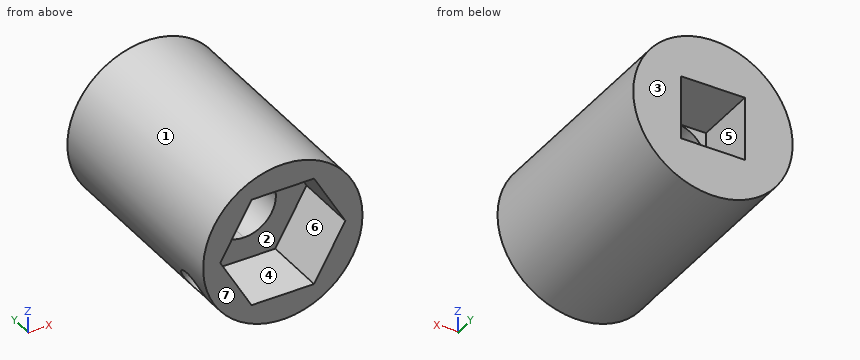
```python
from build123d import *

# Parameters (mm, degrees)
F0_R     = 63.5
F1_DEPTH = 127
F3_DEPTH = 127.001
F4_DEPTH = 50.8
F5_R     = 63.5
F6_DEPTH = 50.8
F7_R     = 13.4769297295
F8_DEPTH = 43.5797324345


with BuildPart() as f1:
    # F0 (on Front) → F1 (new body)
    with BuildSketch(Plane.XZ):
        Circle(F0_R)
    extrude(amount=F1_DEPTH)

    # F2 (on Front) → F3 (cut, through all)
    with BuildSketch(Plane.XZ):
        with BuildLine():
            ThreePointArc((25.4, 0), (17.9605122594, 17.9605122249), (4.89e-08, 25.4))
            ThreePointArc((4.89e-08, 25.4), (-17.9605122127, 17.9605122716), (-25.4, 3.44e-08))
            ThreePointArc((-25.4, 3.44e-08), (-17.9605122437, -17.9605122406), (3.01e-08, -25.4))
            ThreePointArc((3.01e-08, -25.4), (17.9605122528, -17.9605122315), (25.4, 0))
        make_face()
    extrude(amount=F3_DEPTH, mode=Mode.SUBTRACT)

    # F2 (on Front) → F4 (cut)
    with BuildSketch(Plane.XZ):
        with BuildLine():
            Line((4.89e-08, 25.4), (-25.4, 25.4))
            Line((-25.4, 25.4), (-25.4, 3.44e-08))
            ThreePointArc((-25.4, 3.44e-08), (-17.9605122127, 17.9605122716), (4.89e-08, 25.4))
        make_face()
        with BuildLine():
            Line((25.4, 25.4), (4.89e-08, 25.4))
            ThreePointArc((4.89e-08, 25.4), (17.9605122594, 17.9605122249), (25.4, 0))
            Line((25.4, 0), (25.4, 25.4))
        make_face()
        with BuildLine():
            ThreePointArc((25.4, 0), (17.9605122594, 17.9605122249), (4.89e-08, 25.4))
            ThreePointArc((4.89e-08, 25.4), (-17.9605122127, 17.9605122716), (-25.4, 3.44e-08))
            ThreePointArc((-25.4, 3.44e-08), (-17.9605122437, -17.9605122406), (3.01e-08, -25.4))
            ThreePointArc((3.01e-08, -25.4), (17.9605122528, -17.9605122315), (25.4, 0))
        make_face()
        with BuildLine():
            ThreePointArc((3.01e-08, -25.4), (-17.9605122437, -17.9605122406), (-25.4, 3.44e-08))
            Line((-25.4, 3.44e-08), (-25.4, -25.4))
            Line((-25.4, -25.4), (3.01e-08, -25.4))
        make_face()
        with BuildLine():
            Line((25.4, -25.4), (25.4, 0))
            ThreePointArc((25.4, 0), (17.9605122528, -17.9605122315), (3.01e-08, -25.4))
            Line((3.01e-08, -25.4), (25.4, -25.4))
        make_face()
    extrude(amount=F4_DEPTH, mode=Mode.SUBTRACT)

    # F5 (on face) → F6 (join)
    with BuildSketch(Plane.XZ.offset(127)):
        Circle(F5_R)
        Polygon((-49.8413562896, 0), (-24.9206781448, 43.1638807058), (24.9206781448, 43.1638807058), (49.8413562896, 0), (24.9206781448, -43.1638807058), (-24.9206781448, -43.1638807058), align=None, mode=Mode.SUBTRACT)
    extrude(amount=F6_DEPTH)

    # F7 (on face) → F8 (cut, through all)
    with BuildSketch(Plane(origin=(-37.3810172172, 0, -21.5819403529), x_dir=(0, 1, 0), z_dir=(0.8660254038, 0, 0.5))):
        with Locations((-151.6159176826, 0)):
            Circle(F7_R)
    extrude(amount=-F8_DEPTH, mode=Mode.SUBTRACT)


solid = f1.part
```
Build history of the part. All positions in model axes, mm. Face numbers are marked on the shaded views. A direction names the side the tool comes from. Give positions to 0.01 mm unless a question says otherwise; leave off trailing zeros. Loops run counter-clockwise (first coordinate to the right, second up) from the corner with the lowest first, then second, coordinate; pieces in that order, holes last. Notation, with made-up numbers: (13, -23) - (32, -23) arc R23 cw to (32, 5) - close; hole circle Ø3 at (78, -15.5). An arc over 180 degrees is marked (long way). Use a Markdown table: item, result.
(1) Band-saw the part on B-B (x = 11). Give the cut face in (y, z).
Taken from the geometry:
| item | result |
|---|---|
| outline | (-177.8, -62.54) - (0, -62.54) - (0, -25.4) - (-50.8, -25.4) - (-50.8, -22.89) - (-127, -22.89) - (-127, -43.16) - (-177.8, -43.16) - close; (-177.8, 43.16) - (-127, 43.16) - (-127, 22.89) - (-50.8, 22.89) - (-50.8, 25.4) - (0, 25.4) - (0, 62.54) - (-177.8, 62.54) - close |
(2) Band-saw the part on D-D (y = -160.5). Give the cut face in (x, z).
Taken from the geometry:
| item | result |
|---|---|
| outline | (-59.35, -22.57) - (-42.45, -12.81) - (-49.84, 0) - (-24.92, 43.16) - (24.92, 43.16) - (49.84, 0) - (24.92, -43.16) - (-24.92, -43.16) - (-32.31, -30.36) - (-49.22, -40.12) arc R63.5 ccw (long way) to start |
(3) Drop flat-ended pins along their axis: pin 1 Ø12.5 at (x, z) = (-18, -12.5) entering from +Y; pin 2 Ø15 at (x, y) = (9, -23) entering from +Z; pin 3 Ø3 at (y, z) = (-87, -34) entering from +X. Give the stop position or say it passes through.
Taken from the geometry:
| item | result |
|---|---|
| pin 1 | y = -50.8 |
| pin 2 | z = 63.48 |
| pin 3 | x = 54.55 |
(4) Band-saw the part on C-C (y = -93). Give the cut face in (x, z).
Taken from the geometry:
| item | result |
|---|---|
| outline | circle Ø127 at (0, 0); hole circle Ø50.8 at (0, 0) |
(5) Pull direction X, two halves, no side cores. Call the marked faces 1, 2, 3 and 4: +X half, -X half, draft (parallel to the pull), parting line (faces both ways), or undercut.
Taken from the geometry:
| item | result |
|---|---|
| face 1 | parting line |
| face 2 | undercut |
| face 3 | draft |
| face 4 | undercut |
(6) Which spindle directions (+Z, -Z, +X, -X, +Y, -Y) get a long thin tool onto all of the face, cutting with end or side? Do the marked faces 5, 6 and 7. Say none if no direction does.
Taken from the geometry:
| item | result |
|---|---|
| face 5 | +Y |
| face 6 | -Y |
| face 7 | +Z, -Z, +X, -X, -Y |
(7) Wall check: line 1 along Z through (x, y) = (-1.5, -64); line 2 along Y through (x, z) = (17, 31); line 3 along X through (y, z) = (-115, -19). Give the ranges that are in metal, low to high.
Taken from the geometry:
| item | result |
|---|---|
| line 1 | -63.48 to -25.36, 25.36 to 63.48 |
| line 2 | -127 to 0 |
| line 3 | -60.59 to -16.86, 16.86 to 60.59 |
(8) Band-saw the part on A-A (z = 5). Give the cut face in (x, y), and give its area (3 significant figures).
Taken from the geometry:
| item | result |
|---|---|
| outline | (-63.3, -177.8) - (-46.95, -177.8) - (-46.95, -127) - (-24.9, -127) - (-24.9, -50.8) - (-25.4, -50.8) - (-25.4, 0) - (-63.3, 0) - close; (24.9, -127) - (46.95, -127) - (46.95, -177.8) - (63.3, -177.8) - (63.3, 0) - (25.4, 0) - (25.4, -50.8) - (24.9, -50.8) - close |
| area | 11,400 mm2 |
